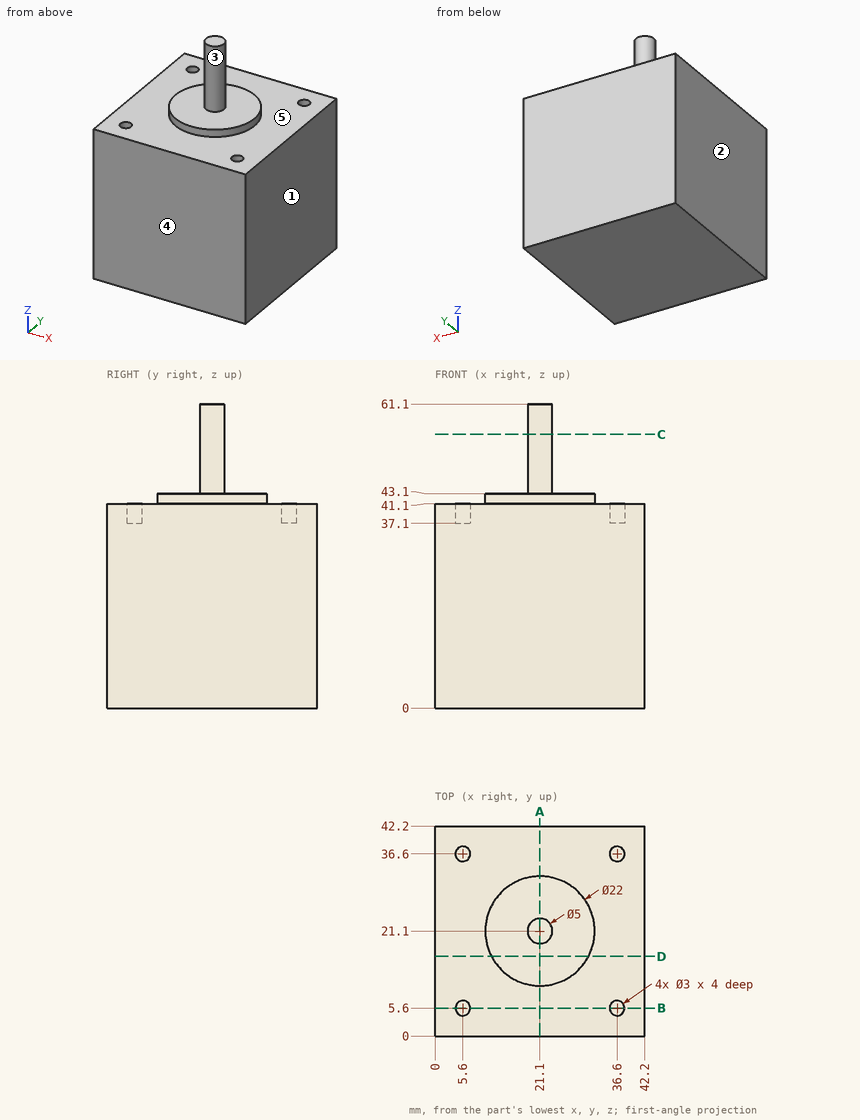
Geometry check sheet. Reference: drawing and pictorial views, mm from the part's lowest x, y, z. A direction names the side the tool comes from. Coordinates: 2 decimals unless noted, no trailing zeros. Write each loop counter-clockwise with the first axis right and the second up, starting at its lowest first coordinate (ties: lowest second). Pieces come first, ordered by that corner, then holes. Notation, with made-up numbers: (69, 0.25) - (73, 0.25) arc R17 cw to (73, 7.25) - close; hole circle Ø6 at (63.25, 64). An arc over 180 degrees is marked (long way). Write item = value, one per line.
Q1. Cross-section at A-A (x = 21.1). Enter the section's corners in (y, z), plus the area to 3 significant figures.
Answer:
outline = (0, 0) - (42.2, 0) - (42.2, 41.1) - (32.1, 41.1) - (32.1, 43.1) - (23.6, 43.1) - (23.6, 61.1) - (18.6, 61.1) - (18.6, 43.1) - (10.1, 43.1) - (10.1, 41.1) - (0, 41.1) - close
area = 1,870 mm²
Q2. Cross-section at C-C (z = 55). Enter the section's corners in (x, y).
Answer:
outline = circle Ø5 at (21.1, 21.1)
Q3. Go/stop test with flat-tipped pins: pin 1 Ø2.5 at (x, y) = (5.6, 36.6) entering from +Z; pin 2 Ø10 at (x, y) = (18, 34) entering from +Z. Record where each tip stops, or that it passes through.
Answer:
pin_1 = 37.1
pin_2 = 43.1
Q4. Cross-section at D-D (y = 16). Enter the section's corners in (x, z).
Answer:
outline = (0, 0) - (42.2, 0) - (42.2, 41.1) - (30.85, 41.1) - (30.85, 43.1) - (11.35, 43.1) - (11.35, 41.1) - (0, 41.1) - close
Q5. Mould release check, pull along X, two halves, no side actions. Record for the marked faces 1, 2 and 3: released by +X, released by -X, zero draft, split by the parting line, or undercut.
Answer:
face_1 = released by +X
face_2 = released by -X
face_3 = split by the parting line
Q6. Access from +Z, -Z, +X, -X, +Y, -Y to the whole of each face (thin tool, end or side, straight path). Record for the marked faces 4 and 5.
Answer:
face_4 = +Z, -Z, +X, -X, -Y
face_5 = +Z
Q7. Cross-section at B-B (y = 5.6). Enter the section's corners in (x, z), plus the area to 3 significant figures.
Answer:
outline = (0, 0) - (42.2, 0) - (42.2, 41.1) - (38.1, 41.1) - (38.1, 37.1) - (35.1, 37.1) - (35.1, 41.1) - (7.1, 41.1) - (7.1, 37.1) - (4.1, 37.1) - (4.1, 41.1) - (0, 41.1) - close
area = 1,710 mm²
Q8. Material ranges on L1, parallel to Y at x = 5.6, z = 38.35; L2, parallel to Y at x = 36, z = 39, recorded low to high. Write a range as from..to.
Answer:
L1 = 0..4.1, 7.1..35.1, 38.1..42.2
L2 = 0..4.23, 6.97..35.23, 37.97..42.2
